The model under review builds one solid part; all positions refer to its coordinate system, in mm. Face numbers are marked on the shaded views. A direction names the side the tool comes from. Round coordinates to 2 decimals unless told otherwise and drop trailing zeros. Loops run counter-clockwise (first coordinate to the right, second up) from the corner with the lowest first, then second, coordinate; pieces in that order, holes last. Notation, with made-up numbers: M 47.5,87.25 L 75.5,87.25 A10 ccw 75.5,104.25 Z; hole C 44,-20 d11. An arc over 180 degrees is marked long. One line per question, with ' | ' between items.
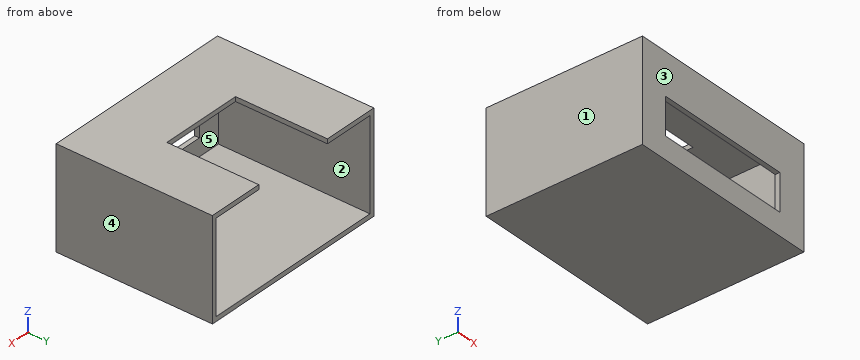
from build123d import *

# Parameters (mm, degrees)
SKETCH6_W           = 201.5
SKETCH6_H           = 99
BOSS_EXTRUDE1_DEPTH = 165
SHELL1_T            = 5
SKETCH7_W           = 150
SKETCH7_H           = 40
CUT_EXTRUDE1_DEPTH  = 165
CUT_EXTRUDE2_REACH  = 287.917
SKETCH8_W           = 90
SKETCH8_H           = 100


with BuildPart() as part:
    # Sketch6 → Boss-Extrude1 (new body)
    with BuildSketch(Plane(origin=(0, 0, 0), x_dir=(1, 0, 0), z_dir=(0, 1, 0))):
        with Locations((100.75, 49.5)):
            Rectangle(SKETCH6_W, SKETCH6_H)
    extrude(amount=BOSS_EXTRUDE1_DEPTH)

    # Shell1
    shell1_openings = [part.faces().sort_by_distance(p)[0] for p in [
        (100.75, 165, -49.5),
    ]]
    offset(amount=SHELL1_T, openings=shell1_openings, kind=Kind.INTERSECTION)

    # Sketch7 → Cut-Extrude1 (cut)
    with BuildSketch(Plane(origin=(0, 0, 0), x_dir=(1, 0, 0), z_dir=(0, 1, 0))):
        with Locations((100, 60)):
            Rectangle(SKETCH7_W, SKETCH7_H)
    extrude(amount=-CUT_EXTRUDE1_DEPTH, mode=Mode.SUBTRACT)

    # Sketch8 → Cut-Extrude2 (cut, up to next)
    with BuildSketch(Plane.XY.offset(5), mode=Mode.PRIVATE) as cut_extrude2_sk1:
        with Locations((100.75, 115)):
            Rectangle(SKETCH8_W, SKETCH8_H)
    cut_extrude2_tool1 = extrude(cut_extrude2_sk1.sketch, amount=-CUT_EXTRUDE2_REACH, mode=Mode.PRIVATE) & part.part
    add(cut_extrude2_tool1.solids().sort_by_distance((100.75, 115, 5))[0], mode=Mode.SUBTRACT)


solid = part.part
1) Machinability: for the marked faces 1 and 2, which of the approach directions +Z, -Z, +X, -X, +Y, -Y give a long, thin tool a straight path to every point of the face, cutting with its end or side? Answer none if there is none.
Output values:
face 1: +Z, -Z, -X, +Y, -Y | face 2: +Y
2) Add section A-A on z = -65.5. State the section outline as (x, y) points, then the cut area to 3 significant figures.
Output values:
outline: M -5,-5 L 25,-5 L 25,0 L 0,0 L 0,165 L -5,165 Z; M 175,-5 L 206.5,-5 L 206.5,165 L 201.5,165 L 201.5,0 L 175,0 Z | area: 1,960 mm²
3) For line 1 (Z direction, x = 53, y = 21); line 2 (X direction, y = 129, z = -15); line 3 (Y direction, x = 138, z = -27.5), list the stretches that pass through material, from the lowest coordinate up.
Output values:
line 1: z = -104 to -99, 0 to 5 | line 2: x = -5 to 0, 201.5 to 206.5 | line 3: y = -5 to 0
4) Insertion check: P1, Ø3, axis at x = 138, z = -14, coming from the +Y side; P2, Ø5.5, axis at x = 107.5, z = 2.5, coming from the +Y side. Each pin has a flat end and moves straight along its axis. Give the tip position at first contact, or say it passes through.
Output values:
P1: stops at y = 0 | P2: stops at y = 65
5) Add section C-C on y = 44.5. State the section outline as (x, z) points, then the cut area to 4 significant figures.
Output values:
outline: M -5,-104 L 206.5,-104 L 206.5,5 L -5,5 Z; hole M 0,-99 L 201.5,-99 L 201.5,0 L 0,0 Z | area: 3,105 mm²
6) Mouldability with a two-part tool opening along X and no side actions: class the marked faces 3, 4 and 5 as +X half, -X half, draft (parallel to the pull), parting line (faces both ways), or undercut.
Output values:
face 3: draft | face 4: +X half | face 5: undercut
7) Add section B-B on x = 141.5. State the section outline as (y, z) points, then the cut area to 4 significant figures.
Output values:
outline: M -5,-104 L 165,-104 L 165,-99 L 0,-99 L 0,-80 L -5,-80 Z; M -5,-40 L 0,-40 L 0,0 L 65,0 L 65,5 L -5,5 Z | area: 1,495 mm²
8) Add section D-D on z = -92. State the section outline as (x, y) points.
Output values:
outline: M -5,-5 L 206.5,-5 L 206.5,165 L 201.5,165 L 201.5,0 L 0,0 L 0,165 L -5,165 Z
